Can you work these out from the model? Positions are in its coordinate system, mm. Face numbers are marked on the shaded views. Give positions to 0.01 mm unless a question says otherwise; leave off trailing zeros. Order: outer loops, then holes, each group sorted by start corner. A loop starts at its lowest first (then second) coordinate and runs counter-clockwise, first axis right, second up. Notation, with made-up numbers: (9.5, 41) - (39.5, 41) arc R30 ccw to (39.5, 80) - close; hole circle Ø8 at (33.25, 39.25). An arc over 180 degrees is marked (long way). Use one line per item in the form item = value. Start each with the question number.
1) Suppose I cut it at B-B, the plane x = 35. Write out the boundary of the cut face in (y, z).
2) Suppose I cut it at A-A, the plane y = -1. Write out the boundary of the cut face in (x, z), and give its area (3 significant figures).
3) Please list where these lines run through material, in increasing order: probe 1 along Z at (x, y) = (-21, -16); probe 2 along Y at (x, z) = (-5, 3.15); probe 3 along X at (y, z) = (-29, 2.65).
4) We'd pull the mould along X, two halves only. Please class the marked faces 1 and 2: released by +X, released by -X, zero draft, split by the parting line, or undercut.
5) For pin 1 (8 mm diameter, centred on x = -27.5, y = 14.5, fed in from +Z); pin 2 (3 mm diameter, centred on x = -18, y = 2, fed in from -Z); pin 3 (6 mm diameter, centred on x = 5, y = -5.5, fed in from -Z), each with a flat end and sliding along its axis, tell me the tip position at first contact or that it passes through.
6) Suppose I cut it at C-C, the plane y = -22. Write out the boundary of the cut face in (x, z).
```python
from build123d import *

# Parameters (mm, degrees)
F1_DEPTH = 2.54
F2_DEPTH = 3.81


with BuildPart() as f1:
    # F0 (on Top) → F1 (new body)
    with BuildSketch(Plane.XY):
        Polygon((41.0611511448, 2.6256455048), (20.5305755724, 38.1856455048), (-20.5305755724, 38.1856455048), (-41.0611511448, 2.6256455048), (-20.5305755724, -32.9343544952), (20.5305755724, -32.9343544952), align=None)
        with BuildLine():
            Line((5.977419205, -17.1863544952), (-5.9265298769, -17.1863544952))
            Line((-5.9265298769, -17.1863544952), (-15.24, 0))
            add(Edge.make_bspline(
                [(-15.24, 0), (-14.825320596, 4.5149536905), (-14.1191885863, 13.7915187507), (0.0347505737, 27.7548005127), (13.7424625985, 13.9441287254), (14.8598540172, 4.6121058638), (15.24, 0)],
                knots=[0, 0, 0, 0, 0.2439742516, 0.5002224701, 0.7539137221, 1, 1, 1, 1], degree=3))
            Line((15.24, 0), (5.977419205, -17.1863544952))
        make_face(mode=Mode.SUBTRACT)
    extrude(amount=F1_DEPTH)

    # F0 (on Top) → F2 (join)
    with BuildSketch(Plane.XY):
        Polygon((43.9940905122, 2.6256455048), (21.9970452561, 40.7256455048), (-21.9970452561, 40.7256455048), (-43.9940905122, 2.6256455048), (-21.9970452561, -35.4743544952), (21.9970452561, -35.4743544952), align=None)
        Polygon((-20.5305755724, 38.1856455048), (20.5305755724, 38.1856455048), (41.0611511448, 2.6256455048), (20.5305755724, -32.9343544952), (-20.5305755724, -32.9343544952), (-41.0611511448, 2.6256455048), align=None, mode=Mode.SUBTRACT)
        with BuildLine():
            Line((-15.24, 0), (-5.9265298769, -17.1863544952))
            Line((-5.9265298769, -17.1863544952), (5.977419205, -17.1863544952))
            Line((5.977419205, -17.1863544952), (15.24, 0))
            add(Edge.make_bspline(
                [(-15.24, 0), (-14.825320596, 4.5149536905), (-14.1191885863, 13.7915187507), (0.0347505737, 27.7548005127), (13.7424625985, 13.9441287254), (14.8598540172, 4.6121058638), (15.24, 0)],
                knots=[0, 0, 0, 0, 0.2439742516, 0.5002224701, 0.7539137221, 1, 1, 1, 1], degree=3))
        make_face()
        with BuildLine():
            Line((-5.08, -14.6463544952), (-12.7, 0))
            add(Edge.make_bspline(
                [(-12.7, 0), (-12.2253034569, 4.5328203475), (-11.3062432336, 13.3088161737), (-3.7440989744, 19.8728472347), (0, 19.8976455048)],
                knots=[0, 0, 0, 0, 0.2577987782, 0.4991243481, 0.4991243481, 0.4991243481, 0.4991243481], degree=3))
            add(Edge.make_bspline(
                [(0, 19.8976455048), (3.7810393885, 19.922688442), (11.7360520972, 13.3740822085), (12.372977607, 4.5371999405), (12.7, 0)],
                knots=[0.4991243481, 0.4991243481, 0.4991243481, 0.4991243481, 0.7428309093, 1, 1, 1, 1], degree=3))
            Line((12.7, 0), (5.08, -14.6463544952))
            Line((5.08, -14.6463544952), (0, -14.6463544952))
            Line((0, -14.6463544952), (-5.08, -14.6463544952))
        make_face(mode=Mode.SUBTRACT)
    extrude(amount=F2_DEPTH)


solid = f1.part
```
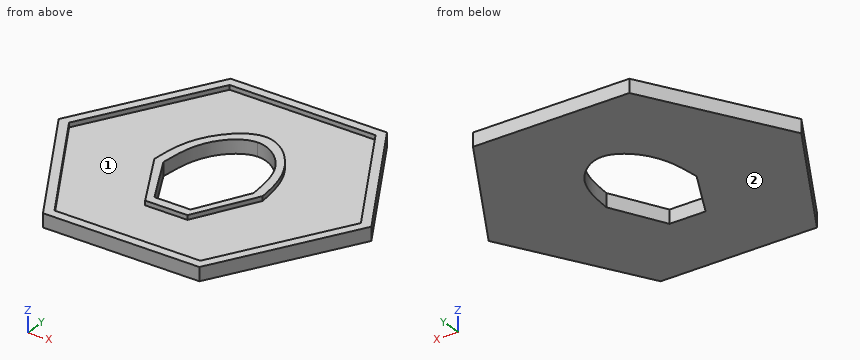
Result sheet:
q1.outline = (-12.95, 0) - (18.2, 0) - (18.2, 3.81) - (13.12, 3.81) - (13.12, 2.54) - (-7.87, 2.54) - (-7.87, 3.81) - (-12.95, 3.81) - close
q2.outline = (-41.9, 0) - (-12.18, 0) - (-12.18, 3.81) - (-14.7, 3.81) - (-14.7, 2.54) - (-38.97, 2.54) - (-38.97, 3.81) - (-41.9, 3.81) - close; (12.18, 0) - (41.9, 0) - (41.9, 3.81) - (38.97, 3.81) - (38.97, 2.54) - (14.7, 2.54) - (14.7, 3.81) - (12.18, 3.81) - close
q2.area = 165 mm²
q3.probe_1 = 0 to 2.54
q3.probe_2 = -35.47 to -32.93, -17.19 to -14.65, 18.1 to 21.45, 38.19 to 40.73
q3.probe_3 = -25.74 to -22.8, 22.8 to 25.74
q4.face_1 = undercut
q4.face_2 = zero draft
q5.pin_1 = 2.54
q5.pin_2 = 0
q5.pin_3 = through
q6.outline = (-29.78, 0) - (29.78, 0) - (29.78, 3.81) - (26.84, 3.81) - (26.84, 2.54) - (-26.84, 2.54) - (-26.84, 3.81) - (-29.78, 3.81) - close
